Geometry: final body of the model. Coordinates: model frame, mm. A direction names the side the tool comes from. Give positions to 0.01 mm unless a question says otherwise; leave off trailing zeros. Write each loop counter-clockwise with the first axis right and the second up, starting at its lowest first coordinate (ties: lowest second). Pieces come first, ordered by that corner, then holes. Notation, with made-up numbers: (87.25, 59.25) -> (104.25, 59.25) arc R9 cw to (104.25, 63.25) -> close; hole circle Ø9 at (10.25, 28). An arc over 180 degrees is marked (long way). Answer as a JSON object with one key per item and string values. Group by question number.
(1) Section query C-C on y = 22.5. Output: boundary loops of the cut face in (x, z).
(2) Section query A-A on x = -24.5. Output: boundary loops of the cut face in (y, z) (3 decimals).
(3) Section query D-D on x = 0. Output: boundary loops of the cut face in (y, z).
(4) Draft query along Y for faces 4 (the face through (0, 7, -6)), 5 (the face through (-22.7, -15, 0)), 6 (the face through (11.444, 5.998, 0.042)), 7 (the face through (33.713, 17.535, 0.084)). Return one class per face: +Y half, -Y half, draft (parallel to the pull), parting line (faces both ways), or undercut.
(5) Material intervals for probe 1 along Y at (x, z) = (0, 3.5); probe 2 along Y at (x, z) = (0, -1.55), sorted ascending.
(6) Set-up query: faces 1 (the face through (7.3, 7.3, -3)), 2 (the face through (-9.76, -2.17, 4.48)), 3 (the face through (31, 17, 6)). Return all of +Z, -Z, +X, -X, +Y, -Y with unobstructed straight access to the full face (end or side cutting, diameter ignored); none if empty.
(7) Contact query for flat-ended pins moving along their axis: pin 1 Ø2 at (x, z) = (18.5, -3) entering from +Y; pin 2 Ø18 at (x, y) = (-13.23, -18.2) entering from -Z; pin 3 Ø4 at (x, z) = (6.5, -2) entering from +Y; pin 4 Ø4 at (x, z) = (-16, -3.5) entering from -Y. Output: stop coordinate, or through.
(8) Section query B-B on z = 4.25. Output: boundary loops of the cut face in (x, y).
Autodesk Inventor part; units mm, degrees
ref_plane "YZ Plane" through (0, 0, 0) normal (1, 0, 0) x (0, 1, 0)
ref_plane "XZ Plane" through (0, 0, 0) normal (0, 1, 0) x (-1, 0, 0)
ref_plane "XY Plane" through (0, 0, 0) normal (0, 0, 1) x (1, 0, 0)
sketch "草圖1" plane through (0, 0, 0) normal (1, 0, 0) x (0, 1, 0)
  line L0 (0, 0) -> (0, 54.3739) construction
  line L1 (0, 0) -> (54.3739, 0) construction
  line L2 (6, 6) -> (6, -6)
  line L3 (38, -6) -> (38, 6)
  line L4 (35, 3) -> (10, 3)
  line L5 (10, 6) -> (10, -6)
  line L6 (10, -3) -> (35, -3)
  line L7 (35, -6) -> (35, 6)
  line L8 (38, 6) -> (35, 6)
  line L9 (10, 6) -> (6, 6)
  line L10 (6, -6) -> (10, -6)
  line L11 (35, -6) -> (38, -6)
  dimension "d2" = 12
  dimension "d3" = 3
  dimension "d4" = 6
  dimension "d5" = 10
  dimension "d6" = 35
  dimension "d7" = 38
  dimension "d8" = 12
revolve "迴轉1" add sketch "草圖1" angle 360 about axis through (0, 0, 0) along (0, 0, 1)
sketch "草圖2" plane through (0, 0, 3) normal (0, 0, 1) x (1, 0, 0)
  circle A0 centre (0, 22.5) radius 10
  point P0 (0, 0)
  dimension "d10" = 20
  dimension "d11" = 22.5
extrude "擠出1" cut sketch "草圖2" against normal through all
pattern_circular "環形陣列1" count 5 over 360 about axis through (0, 0, -10) along (0, 0, 1) of "擠出1"
properties part number "8. 車輪"
Answer list:
{
 "1": {"outline": "(-30.62, -6) -> (-26.81, -6) -> (-26.81, -3) -> (-10, -3) -> (-10, 3) -> (-26.81, 3) -> (-26.81, 6) -> (-30.62, 6) -> close; (10, -3) -> (26.81, -3) -> (26.81, -6) -> (30.62, -6) -> (30.62, 6) -> (26.81, 6) -> (26.81, 3) -> (10, 3) -> close"},
 "2": {"outline": "(-29.047, -6) -> (-24.995, -6) -> (-24.995, -3) -> (-2.554, -3) -> (-2.554, 3) -> (-24.995, 3) -> (-24.995, 6) -> (-29.047, 6) -> close; (16.46, -3) -> (24.995, -3) -> (24.995, -6) -> (29.047, -6) -> (29.047, 6) -> (24.995, 6) -> (24.995, 3) -> (16.46, 3) -> close"},
 "3": {"outline": "(-38, -6) -> (-35, -6) -> (-35, -3) -> (-10, -3) -> (-10, -6) -> (-6, -6) -> (-6, 6) -> (-10, 6) -> (-10, 3) -> (-35, 3) -> (-35, 6) -> (-38, 6) -> close; (6, -6) -> (10, -6) -> (10, -3) -> (12.5, -3) -> (12.5, 3) -> (10, 3) -> (10, 6) -> (6, 6) -> close; (32.5, -3) -> (35, -3) -> (35, -6) -> (38, -6) -> (38, 6) -> (35, 6) -> (35, 3) -> (32.5, 3) -> close"},
 "4": {"face 4": "draft", "face 5": "undercut", "face 6": "undercut", "face 7": "parting line"},
 "5": {"probe 1": "-38 to -35, -10 to -6, 6 to 10, 35 to 38", "probe 2": "-38 to -6, 6 to 12.5, 32.5 to 38"},
 "6": {"face 1": "-Z", "face 2": "+Z", "face 3": "+Z, +X, -X, +Y, -Y"},
 "7": {"pin 1": "y = 33.73", "pin 2": "through", "pin 3": "y = 37.73", "pin 4": "y = -35.33"},
 "8": {"outline": "circle Ø76 at (0, 0); circle Ø20 at (0, 0); hole circle Ø70 at (0, 0); hole circle Ø12 at (0, 0)"}
}
